from build123d import *

# Parameters (mm, degrees)
IZIM1_R                     = 4
Y_KSEKLIK_EKSTR_ZYON1_DEPTH = 5


with BuildPart() as part:
    # Çizim1 → Yükseklik-Ekstrüzyon1 (new body)
    with BuildSketch(Plane.XY):
        with BuildLine():
            Line((-10, 15), (-10, 0))
            ThreePointArc((-10, 0), (0, -10), (10, 0))
            Line((10, 0), (10, 15))
            Line((10, 15), (10, 18))
            Line((10, 18), (-10, 18))
            Line((-10, 18), (-10, 15))
        make_face()
        Circle(IZIM1_R, mode=Mode.SUBTRACT)
    extrude(amount=Y_KSEKLIK_EKSTR_ZYON1_DEPTH)


solid = part.part
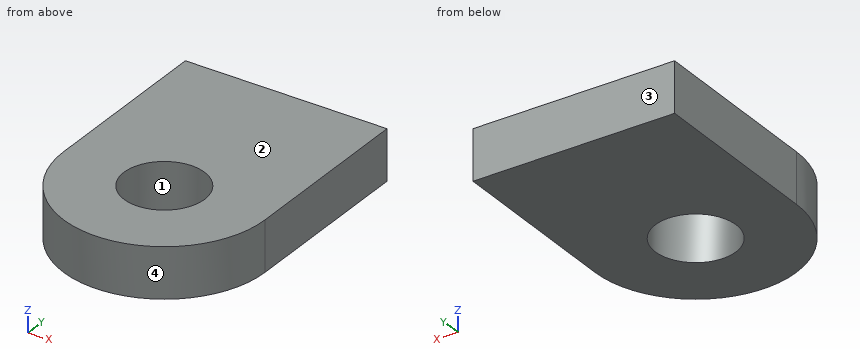
Part model, mm, in its own coordinate system. Face numbers are marked on the shaded views. Coordinates: 2 decimals unless noted, no trailing zeros. Order: outer loops, then holes, each group sorted by start corner. A loop starts at its lowest first (then second) coordinate and runs counter-clockwise, first axis right, second up. Notation, with made-up numbers: M 7.25,53 L 43.25,53 A9 cw 43.25,67 Z; hole C 37.25,11 d10. An arc over 180 degrees is marked long. One line per question, with ' | ' between items.
Q1. Pin check, flat tip, straight feed: P1, Ø2, axis at x = -3.5, z = 2.5, coming from the -Y side. Stop position of the tip, or through.
A:
P1: stops at y = -9.68
Q2. Drill centre lines: line 1 (Y direction, x = 0, z = 3.6); line 2 (X direction, y = 3.25, z = 0.95); line 3 (Y direction, x = 1.25, z = 3.3). Where is each one in solid material? Low to high.
A:
line 1: y = -10 to -4, 4 to 18 | line 2: x = -10 to -2.33, 2.33 to 10 | line 3: y = -9.92 to -3.8, 3.8 to 18
Q3. Slice it at A-A (x = 0). Give the cut face in (y, z).
A:
outline: M -10,0 L -4,0 L -4,5 L -10,5 Z; M 4,0 L 18,0 L 18,5 L 4,5 Z
Q4. Slice it at B-B (y = -3). Give the cut face in (x, z), and give its area (3 significant figures).
A:
outline: M -9.54,0 L -2.65,0 L -2.65,5 L -9.54,5 Z; M 2.65,0 L 9.54,0 L 9.54,5 L 2.65,5 Z | area: 68.9 mm^2
Q5. Slice it at C-C (z = 1.4). Give the cut face in (x, y).
A:
outline: M -10,0 A10 ccw 10,0 L 10,18 L -10,18 Z; hole C 0,0 d8
Q6. Slice it at D-D (x = 5.5). Give the cut face in (y, z), and give its area (3 significant figures).
A:
outline: M -8.35,0 L 18,0 L 18,5 L -8.35,5 Z | area: 132 mm^2
Q7. Two-plate mould, pull along Y, no slides. Class the marked faces 1, 2, 3 and 4: +Y half, -Y half, draft (parallel to the pull), parting line (faces both ways), or undercut.
A:
face 1: undercut | face 2: draft | face 3: +Y half | face 4: -Y half
